from build123d import *

# Parameters (mm, degrees)
SKETCH_1_W             = 60
SKETCH_1_H             = 150
EXTRUDE_1_DEPTH        = 5
SKETCH_2_R             = 1.5
CUT_EXTRUDE_1_DEPTH    = 5
SKETCH_4_R             = 13.55
SKETCH_4_R_2           = 9
CUT_EXTRUDE_1570_DEPTH = 154.05227865
CUT_EXTRUDE_2_DEPTH    = 154.05227865
SKETCH_6_R             = 5
CUT_EXTRUDE_3_DEPTH    = 154.05227865
SKETCH_7_R             = 1.5
CUT_EXTRUDE_4_DEPTH    = 154.05227865
SKETCH_8_R             = 4.5
CUT_EXTRUDE_5_DEPTH    = 2
CUT_EXTRUDE_6_DEPTH    = 154.05227865
FILLET_3_R             = 2
FILLET_4_R             = 5


with BuildPart() as part:
    # 草图1 → 凸台-拉伸1 (new body)
    with BuildSketch(Plane.XY):
        with Locations((0, 75)):
            Rectangle(SKETCH_1_W, SKETCH_1_H)
    extrude(amount=EXTRUDE_1_DEPTH)

    # 草图2 → 切除-拉伸1 (cut)
    with BuildSketch(Plane.XY.offset(5)):
        with BuildLine():
            Line((-20, 4), (-20, 0))
            Line((-20, 0), (20, 0))
            Line((20, 0), (20, 4))
            ThreePointArc((20, 4), (20.707106781, 5.707106781), (19, 5))
            Line((19, 5), (-19, 5))
            ThreePointArc((-19, 5), (-20.707106781, 5.707106781), (-20, 4))
        make_face()
        with Locations((-25, 10)):
            Circle(SKETCH_2_R)
        with Locations((25, 10)):
            Circle(SKETCH_2_R)
        with Locations((8, 9)):
            Circle(SKETCH_2_R)
        with Locations((-8, 9)):
            Circle(SKETCH_2_R)
    extrude(amount=-CUT_EXTRUDE_1_DEPTH, mode=Mode.SUBTRACT)

    # 草图4 → Cut-Extrude 1570 (cut, through all)
    with BuildSketch(Plane.XY.offset(5)):
        with Locations((0, 128)):
            Circle(SKETCH_4_R)
        with Locations((0, 38)):
            Circle(SKETCH_4_R_2)
    extrude(amount=-CUT_EXTRUDE_1570_DEPTH, mode=Mode.SUBTRACT)

    # 草图5 → 切除-拉伸2 (cut, through all)
    with BuildSketch(Plane.XY.offset(5)):
        Polygon((-15, 106.983208217), (-15, 90.349685577), (-30, 77.76319111), (-30, 124.859512106), (-30, 150), (-11.874342087, 150), (-22, 139.874342087), (-25, 136.874342087), (-25, 119.125657913), (-22, 116.125657913), (-15, 109.125657913), align=None)
        Polygon((11.874342087, 150), (30, 131.874342087), (30, 150), align=None)
    extrude(amount=-CUT_EXTRUDE_2_DEPTH, mode=Mode.SUBTRACT)

    # 草图6 → 切除-拉伸3 (cut, through all)
    with BuildSketch(Plane.XY.offset(5)):
        with Locations((0, 83)):
            Circle(SKETCH_6_R)
    extrude(amount=-CUT_EXTRUDE_3_DEPTH, mode=Mode.SUBTRACT)

    # 草图7 → 切除-拉伸4 (cut, through all)
    with BuildSketch(Plane.XY.offset(5)):
        with Locations((18, 136)):
            Circle(SKETCH_7_R)
        with Locations((-18, 136)):
            Circle(SKETCH_7_R)
        with Locations((-18, 120)):
            Circle(SKETCH_7_R)
        with Locations((18, 120)):
            Circle(SKETCH_7_R)
        with Locations((0, 63)):
            Circle(SKETCH_7_R)
        with Locations((0, 103)):
            Circle(SKETCH_7_R)
        with Locations((-18, 46)):
            Circle(SKETCH_7_R)
        with Locations((-18, 30)):
            Circle(SKETCH_7_R)
        with Locations((18, 46)):
            Circle(SKETCH_7_R)
        with Locations((18, 30)):
            Circle(SKETCH_7_R)
    extrude(amount=-CUT_EXTRUDE_4_DEPTH, mode=Mode.SUBTRACT)

    # 草图8 → 切除-拉伸5 (cut)
    with BuildSketch(Plane(origin=(0, 0, 0), x_dir=(-1, 0, 0), z_dir=(0, 0, -1))):
        with Locations((-18, 136)):
            Circle(SKETCH_8_R)
        with Locations((18, 136)):
            Circle(SKETCH_8_R)
        with Locations((-18, 120)):
            Circle(SKETCH_8_R)
        with Locations((18, 120)):
            Circle(SKETCH_8_R)
        with Locations((0, 103)):
            Circle(SKETCH_8_R)
        with Locations((0, 63)):
            Circle(SKETCH_8_R)
    extrude(amount=-CUT_EXTRUDE_5_DEPTH, mode=Mode.SUBTRACT)

    # 草图9 → 切除-拉伸6 (cut, through all)
    with BuildSketch(Plane.XY.offset(5)):
        Polygon((-23, 58.183667551), (-14.257978987, 81.83446411), (-23, 74.499037502), align=None)
        with BuildLine():
            ThreePointArc((-6, 75), (-7.735015794, 76.662056275), (-9.023511491, 78.689983716))
            Line((-9.023511491, 78.689983716), (-18.086264707, 54.171473379))
            Line((-18.086264707, 54.171473379), (-6, 65.586278935))
            Line((-6, 65.586278935), (-6, 75))
        make_face()
        with BuildLine():
            ThreePointArc((7.893692694, 76.860813111), (7.008875126, 75.867281761), (6, 75))
            Line((6, 75), (6, 65.586278935))
            Line((6, 65.586278935), (17.467722447, 54.75565218))
            Line((17.467722447, 54.75565218), (7.893692694, 76.860813111))
        make_face()
        Polygon((23, 92.975167824), (11.96629434, 82.554445812), (12.398973079, 81.555448171), (23, 57.079087413), align=None)
        with BuildLine():
            Line((23, 115.093785686), (-0.401978174, 92.991917411))
            ThreePointArc((-0.401978174, 92.991917411), (4.47705407, 91.941811162), (8.240956067, 88.664507313))
            Line((8.240956067, 88.664507313), (23, 102.60360436))
            Line((23, 102.60360436), (23, 115.093785686))
        make_face()
    extrude(amount=-CUT_EXTRUDE_6_DEPTH, mode=Mode.SUBTRACT)

    # 圆角3
    # the kernel refuses this fillet: 2 mm, written as the material it adds along each edge
    with BuildSketch(Plane(origin=(-9.023511491, 78.689983716, 5), x_dir=(-0.34670280320630176, -0.9379750349816846, 0), z_dir=(0, 0, -1))) as fillet_3_piece_1:
        with BuildLine():
            CenterArc((3.751460465, -2), FILLET_3_R, 90, 114.464402838)
            ThreePointArc((1.931022987, -2.82825563), (1.087482709, -1.330850611), (0, 0))
            Line((0, 0), (3.751460465, 0))
        make_face()
    extrude(amount=5)
    with BuildSketch(Plane(origin=(-6, 75, 5), x_dir=(-0.7733966621340284, 0.6339223950926041, 0), z_dir=(0, 0, -1))) as fillet_3_piece_2:
        with BuildLine():
            CenterArc((0.948198213, -1.998141534), FILLET_3_R, 92.470208625, 48.189685104)
            Line((-0.598595111, -0.730296743), (0, 0))
            ThreePointArc((0, 0), (0.430999188, -0.009292332), (0.861998376, 0))
        make_face()
    extrude(amount=5)
    with BuildSketch(Plane(origin=(-6, 65.586278935, 5), x_dir=(0, 1, 0), z_dir=(0, 0, -1)), Plane(origin=(6, 65.586278935, 5), x_dir=(0.7270131525498171, -0.6866235329637167, 0), z_dir=(0, 0, -1))) as fillet_3_piece_3:
        with BuildLine():
            CenterArc((FILLET_3_R * 0.431046489238, -FILLET_3_R), FILLET_3_R, 90, 46.636577042)
            Line((-FILLET_3_R * 0.295966663312, -FILLET_3_R * 0.313376467036), (0, 0))
            Line((0, 0), (FILLET_3_R * 0.431046489238, 0))
        make_face()
    extrude(amount=5)
    with BuildSketch(Plane(origin=(-18.086264707, 54.171473379, 5), x_dir=(0.3467028032063488, 0.9379750349816672, 0), z_dir=(0, 0, -1))) as fillet_3_piece_4:
        with BuildLine():
            CenterArc((FILLET_3_R * 4.2717705967, FILLET_3_R), FILLET_3_R, 116.350801131, 153.649198869)
            Line((FILLET_3_R * 3.82790471313, FILLET_3_R * 1.89609323031), (0, 0))
            Line((0, 0), (FILLET_3_R * 4.2717705967, 0))
        make_face()
    extrude(amount=5)
    with BuildSketch(Plane(origin=(6, 75, 5), x_dir=(0, -1, 0), z_dir=(0, 0, -1))) as fillet_3_piece_5:
        with BuildLine():
            CenterArc((0.94427191, -2), FILLET_3_R, 90, 48.189685104)
            ThreePointArc((-0.546440075, -0.666666667), (-0.266033379, -0.339223951), (0, 0))
            Line((0, 0), (0.94427191, 0))
        make_face()
    extrude(amount=5)
    with BuildSketch(Plane(origin=(7.893692694, 76.860813111, 5), x_dir=(0.39743711176533947, -0.9176294144106459, 0), z_dir=(0, 0, -1))) as fillet_3_piece_6:
        with BuildLine():
            CenterArc((2.897165869, 2), FILLET_3_R, 166.489199346, 103.510800654)
            ThreePointArc((0.952514075, 2.467257316), (0.558182396, 1.202000398), (0, 0))
            Line((0, 0), (2.897165869, 0))
        make_face()
    extrude(amount=5)
    with BuildSketch(Plane(origin=(17.467722447, 54.75565218, 5), x_dir=(-0.39743711176536367, 0.9176294144106355, 0), z_dir=(0, 0, -1))) as fillet_3_piece_7:
        with BuildLine():
            CenterArc((FILLET_3_R * 4.86762612827, -FILLET_3_R), FILLET_3_R, 90, 156.781480378)
            Line((FILLET_3_R * 4.47338714864, -FILLET_3_R * 1.91900795804), (0, 0))
            Line((0, 0), (FILLET_3_R * 4.86762612827, 0))
        make_face()
    extrude(amount=5)
    with BuildSketch(Plane(origin=(8.240956067, 88.664507313, 5), x_dir=(0.7270131525498188, 0.6866235329637153, 0), z_dir=(0, 0, -1))) as fillet_3_piece_8:
        with BuildLine():
            CenterArc((2.110522706, -2), FILLET_3_R, 90, 87.804380429)
            ThreePointArc((0.111991009, -1.923377175), (0.102424036, -0.958985229), (0, 0))
            Line((0, 0), (2.110522706, 0))
        make_face()
    extrude(amount=5)
    with BuildSketch(Plane(origin=(-0.401978174, 92.991917411, 5), x_dir=(0.9892255370424882, -0.14639957944953544, 0), z_dir=(0, 0, -1))) as fillet_3_piece_9:
        with BuildLine():
            CenterArc((4.09301108, -1.965082086), FILLET_3_R, 100.722120143, 117.496122758)
            Line((2.521691174, -3.202399246), (0, 0))
            ThreePointArc((0, 0), (1.860459582, -0.174589569), (3.720919164, 0))
        make_face()
    extrude(amount=5)
    with BuildSketch(Plane(origin=(23, 115.093785686, 5), x_dir=(-0.7270131525498174, -0.6866235329637166, 0), z_dir=(0, 0, -1))) as fillet_3_piece_10:
        with BuildLine():
            CenterArc((FILLET_3_R * 2.31993537813, -FILLET_3_R), FILLET_3_R, 90, 133.363422958)
            Line((FILLET_3_R * 1.59292222558, -FILLET_3_R * 1.68662353296), (0, 0))
            Line((0, 0), (FILLET_3_R * 2.31993537813, 0))
        make_face()
    extrude(amount=5)
    with BuildSketch(Plane(origin=(23, 102.60360436, 5), x_dir=(-0.7270131525498177, -0.6866235329637163, 0), z_dir=(0, 0, -1))) as fillet_3_piece_11:
        with BuildLine():
            CenterArc((FILLET_3_R * 0.431046489238, FILLET_3_R), FILLET_3_R, 223.363422958, 46.636577042)
            Line((-FILLET_3_R * 0.295966663312, FILLET_3_R * 0.313376467036), (0, 0))
            Line((0, 0), (FILLET_3_R * 0.431046489238, 0))
        make_face()
    extrude(amount=5)
    with BuildSketch(Plane(origin=(23, 57.079087413, 5), x_dir=(0, 1, 0), z_dir=(0, 0, -1))) as fillet_3_piece_12:
        with BuildLine():
            CenterArc((FILLET_3_R * 4.82498830039, -FILLET_3_R), FILLET_3_R, 90, 156.58194258)
            Line((FILLET_3_R * 4.42755118863, -FILLET_3_R * 1.91762941441), (0, 0))
            Line((0, 0), (FILLET_3_R * 4.82498830039, 0))
        make_face()
    extrude(amount=5)
    with BuildSketch(Plane(origin=(11.96629434, 82.554445812, 5), x_dir=(0.3974371117653669, -0.917629414410634, 0), z_dir=(0, 0, -1))) as fillet_3_piece_13:
        with BuildLine():
            CenterArc((FILLET_3_R * 0.700918309769, -FILLET_3_R), FILLET_3_R, 90, 70.054634461)
            Line((-FILLET_3_R * 0.239100017486, -FILLET_3_R * 0.658876057091), (0, 0))
            Line((0, 0), (FILLET_3_R * 0.700918309769, 0))
        make_face()
    extrude(amount=5)
    with BuildSketch(Plane(origin=(23, 92.975167824, 5), x_dir=(0, -1, 0), z_dir=(0, 0, -1))) as fillet_3_piece_14:
        with BuildLine():
            CenterArc((FILLET_3_R * 2.31993537813, FILLET_3_R), FILLET_3_R, 136.636577042, 133.363422958)
            Line((FILLET_3_R * 1.59292222558, FILLET_3_R * 1.68662353296), (0, 0))
            Line((0, 0), (FILLET_3_R * 2.31993537813, 0))
        make_face()
    extrude(amount=5)
    with BuildSketch(Plane(origin=(-14.257978987, 81.83446411, 5), x_dir=(-0.34670280320634744, -0.9379750349816677, 0), z_dir=(0, 0, -1))) as fillet_3_piece_15:
        with BuildLine():
            CenterArc((FILLET_3_R * 3.76962956743, FILLET_3_R), FILLET_3_R, 119.71422409, 150.28577591)
            Line((FILLET_3_R * 3.27395527024, FILLET_3_R * 1.86850848649), (0, 0))
            Line((0, 0), (FILLET_3_R * 3.76962956743, 0))
        make_face()
    extrude(amount=5)
    with BuildSketch(Plane(origin=(-23, 58.183667551, 5), x_dir=(0.34670280320634733, 0.9379750349816677, 0), z_dir=(0, 0, -1))) as fillet_3_piece_16:
        with BuildLine():
            CenterArc((FILLET_3_R * 5.58972992736, -FILLET_3_R), FILLET_3_R, 90, 159.71422409)
            Line((FILLET_3_R * 5.24302712415, -FILLET_3_R * 1.93797503498), (0, 0))
            Line((0, 0), (FILLET_3_R * 5.58972992736, 0))
        make_face()
    extrude(amount=5)
    with BuildSketch(Plane(origin=(-23, 74.499037502, 5), x_dir=(0, -1, 0), z_dir=(0, 0, -1))) as fillet_3_piece_17:
        with BuildLine():
            CenterArc((FILLET_3_R * 0.466307658155, -FILLET_3_R), FILLET_3_R, 90, 50)
            Line((-FILLET_3_R * 0.299736784964, -FILLET_3_R * 0.357212390313), (0, 0))
            Line((0, 0), (FILLET_3_R * 0.466307658155, 0))
        make_face()
    extrude(amount=5)

    # 圆角4
    fillet_4_edges = [part.edges().sort_by_distance(p)[0] for p in [
        (-11.874342087, 150, 2.5),
        (-25, 136.874342087, 2.5),
        (30, 0, 2.5),
        (-25, 119.125657913, 2.5),
        (-15, 109.125657913, 2.5),
        (-30, 0, 2.5),
        (-15, 90.349685577, 2.5),
        (-30, 77.76319111, 2.5),
        (11.874342087, 150, 2.5),
        (30, 131.874342087, 2.5),
    ]]
    fillet(fillet_4_edges, radius=FILLET_4_R)


solid = part.part
Input: part model. Units: mm. Frame: model coordinates. A direction names the side the tool comes from. Coordinates: 2 decimals unless noted, no trailing zeros. Order: outer loops, then holes, each group sorted by start corner. A loop starts at its lowest first (then second) coordinate and runs counter-clockwise, first axis right, second up. Notation, with made-up numbers: M 87,-25.5 L 108,-25.5 A20 cw 108,0.5 Z; hole C -4,69.5 d10. An arc over 180 degrees is marked long. Write item = value, one per line. Start each with the question number.
(1) Pull-direction query (X, two-part tool) for faces 4 (the flat face through (0, 57, 0)), 5 (the flat face through (11.21, 103.96, 2.54)), 6 (the flat face through (30, 67, 2)); classes: released by +X, released by -X, zero draft, split by the parting line, or undercut.
(2) Section A-A on y = 38. Output: boundary loops of the cut face in (x, z).
(3) Reachability of faces 1 (the flat face through (-20, 120, 2)), 2 (the cylindrical face through (21.762, 112.303, 2.535)), 3 (the cylindrical face through (-29.544, 77.517, 2.465)) from +Z, -Z, +X, -X, +Y, -Y: full face, straight path, thin tool, end or side. Return the list, or none.
(4) First-contact query: P1, Ø2.5, axis at y = 78, z = 1.5, coming from the -X side; P2, Ø2, axis at x = 3.5, z = 3, coming from the -Y side; P3, Ø1.5, axis at x = 19.5, z = 0.5, coming from the +Y side. Flat tips, straight axial feed; report the tip coordinate or a pass-through.
(5) Line query: line 1 along Y through (x, z) = (0, 3.75); line 2 along X through (y, z) = (139, 0.65); line 3 along Y through (x, z) = (14.5, 3.55). Output: solid intervals per line, ascending. Write a range as [from, to].
(6) Section B-B on z = 3.6. Give the number of separate pieces and of enclosed holes in the cut face, and give its area (3 significant figures).
Result set:
q1.face_4 = zero draft
q1.face_5 = undercut
q1.face_6 = released by +X
q2.outline = M -30,0 L -9,0 L -9,5 L -30,5 Z; M 9,0 L 30,0 L 30,5 L 9,5 Z
q3.face_1 = -Z
q3.face_2 = +Z, -Z
q3.face_3 = +Z, -Z, -X, +Y
q4.P1 = -29.82
q4.P2 = 5
q4.P3 = 143.12
q5.line_1 = [5, 29], [47, 61.5], [64.5, 78], [88, 101.5], [104.5, 114.45], [141.55, 150]
q5.line_2 = [-22.87, -21.35], [-14.65, -7.91], [7.91, 14.65], [21.35, 22.87]
q5.line_3 = [5, 76.7], [84.95, 94.58], [107.07, 147.37]
q6.separate_pieces = 1
q6.enclosed_holes = 22
q6.area = 6,280 mm²
